from build123d import *

# Parameters (mm, degrees)
BASE_FLANGE1_DEPTH = 25
CHAMFER1_SIZE      = 5
SKETCH7_R          = 11.05
SKETCH7_R_2        = 1.75
CUT_EXTRUDE1_DEPTH = 78.685262438
CUT_EXTRUDE2_DEPTH = 78.685262438


# Sheet-metal steps are written as plain solids
with BuildPart() as part:
    # Sketch2 → Base-Flange1 (new, symmetric)
    with BuildSketch(Plane(origin=(0, 0, 0), x_dir=(1, 0, 0), z_dir=(0, 1, 0))):
        with BuildLine():
            Line((0, 51), (0, 6.5))
            ThreePointArc((0, 6.5), (-1.903805922, 1.903805922), (-6.5, 0))
            Line((-6.5, 0), (-53, 0))
            Line((-53, 0), (-53, 3))
            Line((-53, 3), (-6.5, 3))
            ThreePointArc((-6.5, 3), (-4.025126266, 4.025126266), (-3, 6.5))
            Line((-3, 6.5), (-3, 51))
            Line((-3, 51), (0, 51))
        make_face()
    extrude(amount=BASE_FLANGE1_DEPTH, both=True)

    # Chamfer1
    chamfer1_edges = [part.edges().sort_by_distance(p)[0] for p in [
        (-1.5, 25, -51),
        (-53, 25, -1.5),
        (-1.5, -25, -51),
        (-53, -25, -1.5),
    ]]
    chamfer(chamfer1_edges, length=CHAMFER1_SIZE)

    # Sketch7 → Cut-Extrude1 (cut, through all)
    with BuildSketch(Plane(origin=(0, 0, 0), x_dir=(0, 0, -1), z_dir=(1, 0, 0))):
        with Locations((30, 0)):
            Circle(SKETCH7_R)
        with Locations((45.5, 15.5)):
            Circle(SKETCH7_R_2)
        with Locations((14.5, 15.5)):
            Circle(SKETCH7_R_2)
        with Locations((14.5, -15.5)):
            Circle(SKETCH7_R_2)
        with Locations((45.5, -15.5)):
            Circle(SKETCH7_R_2)
    extrude(amount=-CUT_EXTRUDE1_DEPTH, mode=Mode.SUBTRACT)

    # Sketch8 → Cut-Extrude2 (cut, through all)
    with BuildSketch(Plane.XY):
        with BuildLine():
            Line((-42, 17.1), (-12, 17.1))
            ThreePointArc((-12, 17.1), (-9.9, 15), (-12, 12.9))
            Line((-12, 12.9), (-42, 12.9))
            ThreePointArc((-42, 12.9), (-44.1, 15), (-42, 17.1))
        make_face()
        with BuildLine():
            Line((-42, -17.1), (-12, -17.1))
            ThreePointArc((-12, -17.1), (-9.9, -15), (-12, -12.9))
            Line((-12, -12.9), (-42, -12.9))
            ThreePointArc((-42, -12.9), (-44.1, -15), (-42, -17.1))
        make_face()
    extrude(amount=-CUT_EXTRUDE2_DEPTH, mode=Mode.SUBTRACT)


solid = part.part
Geometry check sheet. Reference: the model listing, model coordinates, mm. A direction names the side the tool comes from. Give positions to 0.01 mm unless a question says otherwise; leave off trailing zeros. Loops run counter-clockwise (first coordinate to the right, second up) from the corner with the lowest first, then second, coordinate; pieces in that order, holes last.
(1) Section check D-D on z = -38. Record the cut outline in (x, y), then the cut area to 3 significant figures.
From the geometry:
outline: (-3, -25) - (0, -25) - (0, -7.62) - (-3, -7.62) - close; (-3, 7.62) - (0, 7.62) - (0, 25) - (-3, 25) - close
area: 104 mm2
(2) Set-up check for faces 4 (the flat face through (0, -5, -19)), 5 (the flat face through (-3, 0.4, -18.5)), 6 (the flat face through (-27, -12.9, -1)): record each of +Z, -Z, +X, -X, +Y, -Y from which the full face is reachable in a straight line by a thin tool's end or side.
From the geometry:
face 4: +Z, -Z, +X, +Y, -Y
face 5: -Z, -X, +Y, -Y
face 6: +Z, -Z
(3) Depth check by flat-ended pin: pin 1 Ø4 at (x, y) = (-28, 18.5) entering from -Z; pin 2 Ø4.5 at (y, z) = (-15.5, -14.5) entering from -X; pin 3 Ø2 at (y, z) = (15.5, -14.5) entering from -X. Enter the tip coordinate at first touch or a pass-through.
From the geometry:
pin 1: stops at z = -3
pin 2: stops at x = -3
pin 3: passes through
(4) Section check A-A on x = -32.5. Record the cut outline in (y, z), then the cut area to 3 significant figures.
From the geometry:
outline: (-25, -3) - (-17.1, -3) - (-17.1, 0) - (-25, 0) - close; (-12.9, -3) - (12.9, -3) - (12.9, 0) - (-12.9, 0) - close; (17.1, -3) - (25, -3) - (25, 0) - (17.1, 0) - close
area: 125 mm2
(5) Section check C-C on y = 21. Record the cut outline in (x, z), then the cut area to 3 significant figures.
From the geometry:
outline: (-52, -3) - (-6.5, -3) arc R3.5 cw to (-3, -6.5) - (-3, -50) - (0, -50) - (0, -6.5) arc R6.5 ccw to (-6.5, 0) - (-52, 0) - close
area: 291 mm2
(6) Release check for a two-part mould opening along Z. For faces 1 (the cylindrical face through (-1.479, 16.026, -47.169)), 2 (the flat face through (-30, 0, -3)), 3 (the cylindrical face through (-9.9, -15, -1.5)) record: released by +Z, released by -Z, zero draft, split by the parting line, or undercut.
From the geometry:
face 1: undercut
face 2: released by -Z
face 3: zero draft
(7) Thickness scan on L1, parallel to Y at x = -2, z = -45.5; L2, parallel to Z at x = -1, y = 15; L3, parallel to Y at x = -1, z = -30. Record the ranges inside material, lowest first.
From the geometry:
L1: y = -25 to -17.25, -13.75 to 13.75, 17.25 to 25
L2: z = -51 to -47.18, -43.82 to -16.18, -12.82 to -3.04
L3: y = -25 to -11.05, 11.05 to 25
(8) Section check B-B on y = 5. Record the cut outline in (x, z), then the cut area to 3 significant figures.
From the geometry:
outline: (-53, -3) - (-6.5, -3) arc R3.5 cw to (-3, -6.5) - (-3, -20.15) - (0, -20.15) - (0, -6.5) arc R6.5 ccw to (-6.5, 0) - (-53, 0) - close; (-3, -51) - (0, -51) - (0, -39.85) - (-3, -39.85) - close
area: 237 mm2
